Model file for the job. Use its own axes, mm. A direction names the side the tool comes from. Coordinates: 2 decimals unless noted, no trailing zeros. Loops run counter-clockwise (first coordinate to the right, second up) from the corner with the lowest first, then second, coordinate; pieces in that order, holes last.
from build123d import *

# Parameters (mm, degrees)
SKETCH1_R               = 15
BOSS_EXTRUDE1_DEPTH     = 40
CUT_EXTRUDE1_DEPTH      = 15
SKETCH3_R               = 2
CUT_EXTRUDE2_DEPTH      = 15
CUT_EXTRUDE3_DEPTH      = 9
SKETCH5_R               = 2.5
CUT_EXTRUDE4_DEPTH      = 19.550000101
CUT_EXTRUDE4_DEPTH_BACK = 12.4500001


with BuildPart() as part:
    # Sketch1 → Boss-Extrude1 (new body)
    with BuildSketch(Plane(origin=(0, 0, 0), x_dir=(1, 0, 0), z_dir=(0, 1, 0))):
        Circle(SKETCH1_R)
    extrude(amount=BOSS_EXTRUDE1_DEPTH)

    # Sketch2 → Cut-Extrude1 (cut)
    with BuildSketch(Plane.XZ):
        with BuildLine():
            Line((-4.000002932, 5), (3.999997068, 5))
            add(Edge.make_bspline(
                [(3.999997068, 5), (8.199974497, 0.009249301), (3.999997068, -5)],
                knots=[0, 0, 0, 1, 1, 1], degree=2))
            Line((3.999997068, -5), (-4.000002932, -5))
            add(Edge.make_bspline(
                [(-4.000002932, 5), (-8.199982148, -0.00561634), (-4.000002932, -5)],
                knots=[0, 0, 0, 1, 1, 1], degree=2))
        make_face()
    extrude(amount=-CUT_EXTRUDE1_DEPTH, mode=Mode.SUBTRACT)

    # Sketch3 → Cut-Extrude2 (cut)
    with BuildSketch(Plane.XY.offset(-5)):
        with Locations((0, 12.004234523)):
            Circle(SKETCH3_R)
    extrude(amount=-CUT_EXTRUDE2_DEPTH, mode=Mode.SUBTRACT)

    # Sketch4 → Cut-Extrude3 (cut)
    with BuildSketch(Plane(origin=(0, 40, 0), x_dir=(1, 0, 0), z_dir=(0, 1, 0))):
        with BuildLine():
            Line((-5, 3.55), (5, 3.55))
            add(Edge.make_bspline(
                [(5, 3.55), (5.491620402, 0), (5, -3.55)],
                knots=[0, 0, 0, 1, 1, 1], degree=2))
            Line((5, -3.55), (-5, -3.55))
            add(Edge.make_bspline(
                [(-5, 3.55), (-5.491620402, 0), (-5, -3.55)],
                knots=[0, 0, 0, 1, 1, 1], degree=2))
        make_face()
    extrude(amount=-CUT_EXTRUDE3_DEPTH, mode=Mode.SUBTRACT)

    # Sketch5 → Cut-Extrude4 (cut, two sides)
    with BuildSketch(Plane(origin=(0, 0, 3.55), x_dir=(-1, 0, 0), z_dir=(0, 0, -1))) as cut_extrude4_sk:
        with Locations((0, 36)):
            Circle(SKETCH5_R)
    extrude(amount=CUT_EXTRUDE4_DEPTH, mode=Mode.SUBTRACT)
    extrude(cut_extrude4_sk.sketch, amount=-CUT_EXTRUDE4_DEPTH_BACK, mode=Mode.SUBTRACT)


solid = part.part
Q1. Slice it at B-B (z = -8.5). List the corners of the cut face in (x, y).
Answers:
outline: (-12.36, 0) - (12.36, 0) - (12.36, 40) - (-12.36, 40) - close; hole circle Ø5 at (0, 36); hole circle Ø4 at (0, 12)
Q2. Drill centre lines: line 1 (Y direction, x = 0, z = -9); line 2 (Y direction, x = 0, z = 9.75); line 3 (Y direction, x = 3.5, z = 1). Where is each one in solid material? Low to high.
Answers:
line 1: y = 0 to 10, 14 to 33.5, 38.5 to 40
line 2: y = 0 to 33.5, 38.5 to 40
line 3: y = 15 to 31
Q3. Which spindle directions (+Z, -Z, +X, -X, +Y, -Y) get a long thin tool onto all of the face, cutting with end or side? Do faces 1 (the flat face through (0, 7, -5)), 2 (the cylindrical face through (0.54, 33.56, -9.2)), 3 (the flat face through (0, 31, 0)), 4 (the cylindrical face through (-0.26, 13.987, -9.932)). Say none if no direction does.
Answers:
face 1: -Y
face 2: +Z, -Z
face 3: +Y
face 4: -Z
Q4. Slice it at C-C (y = 23). List the corners of the cut face in (x, z).
Answers:
outline: circle Ø30 at (0, 0)
Q5. Slice it at A-A (x = 0). List the corners of the cut face in (y, z), and give its area (3 significant figures).
Answers:
outline: (0, -15) - (10, -15) - (10, -5) - (0, -5) - close; (0, 5) - (15, 5) - (15, -5) - (14, -5) - (14, -15) - (33.5, -15) - (33.5, -3.55) - (31, -3.55) - (31, 3.55) - (33.5, 3.55) - (33.5, 15) - (0, 15) - close; (38.5, -15) - (40, -15) - (40, -3.55) - (38.5, -3.55) - close; (38.5, 3.55) - (40, 3.55) - (40, 15) - (38.5, 15) - close
area: 832 mm2
Q6. Mould opens along Z. For faces 5 (the flat face through (0, 7, 5)), 6 (the flat face through (6, 40, 0)), 7 (the cylindrical face through (-3.252, 19.72, 14.643)) say: +Z half, -Z half, draft (parallel to the pull), parting line (faces both ways), or undercut.
Answers:
face 5: undercut
face 6: draft
face 7: parting line
Q7. Flat gauge pins, fed straight in: P1, Ø10, axis at x = 2, y = 35.5, coming from the -Z side; P2, Ø6, axis at x = 10.5, y = 15.5, coming from the +Z side; P3, Ø5.5, axis at x = 2, z = -0.5, coming from the +Y side; P4, Ø10, axis at x = 7.5, y = 6.5, coming from the +Z side. Where does each tip first touch, or does it go through?
Answers:
P1: stops at z = -15
P2: stops at z = 12.99
P3: stops at y = 31
P4: stops at z = 14.79
Q8. Slice it at D-D (z = 7). List the corners of the cut face in (x, y).
Answers:
outline: (-13.27, 0) - (13.27, 0) - (13.27, 40) - (-13.27, 40) - close; hole circle Ø5 at (0, 36)
